The drawing under review shows one solid part. Ordinate dimensions are in mm from its lowest x, y, z. A direction names the side the tool comes from. Give positions to 0.01 mm unless a question says otherwise; leave off trailing zeros. Order: outer loops, then holes, each group sorted by start corner. A loop starts at its lowest first (then second) coordinate and runs counter-clockwise, first axis right, second up. Notation, with made-up numbers: (88, 46.25) -> (110, 46.25) arc R20 cw to (110, 68.25) -> close; hole circle Ø3 at (-24, 78). An arc over 180 degrees is marked (long way). Return JSON: item names as keys, results as strings. Group by question number.
1) The part is to be moulded in two halves that separate along X. For the marked faces 3, 4, 5 and 6, say which applies: released by +X, released by -X, zero draft, split by the parting line, or undercut.
2) Add section A-A (x = 67.5). Give the boundary of the cut face in (y, z).
3) Add section B-B (z = 15). Give the boundary of the cut face in (x, y), then the cut area to 3 significant figures.
4) Add section D-D (z = 40). Give the boundary of the cut face in (x, y).
5) Insertion check: P1, Ø24, axis at x = 47.5, z = 28, coming from the -Y side; P2, Ø3, axis at x = 52.5, y = 20, coming from the +Z side; P3, Ø12, axis at x = 25.5, y = 46.5, coming from the +Z side. Each pin has a flat end and moves straight along its axis. Give the tip position at first contact, or say it passes through.
6) Add section C-C (y = 20). Give the boundary of the cut face in (x, z).
7) For the marked faces 1 and 2, list the 3-axis set-ups (+Z, -Z, +X, -X, +Y, -Y) from which the entire face can be reached by the end or side of a thin tool; tool diameter is ignored.
8) To check wall thickness, follow line 1 along X through (y, z) = (50.5, 38.5); line 2 along Y through (x, z) = (67.5, 0.4); line 3 along Z through (x, y) = (5.5, 55). State the ranges of each line that lie inside material, in increasing order.
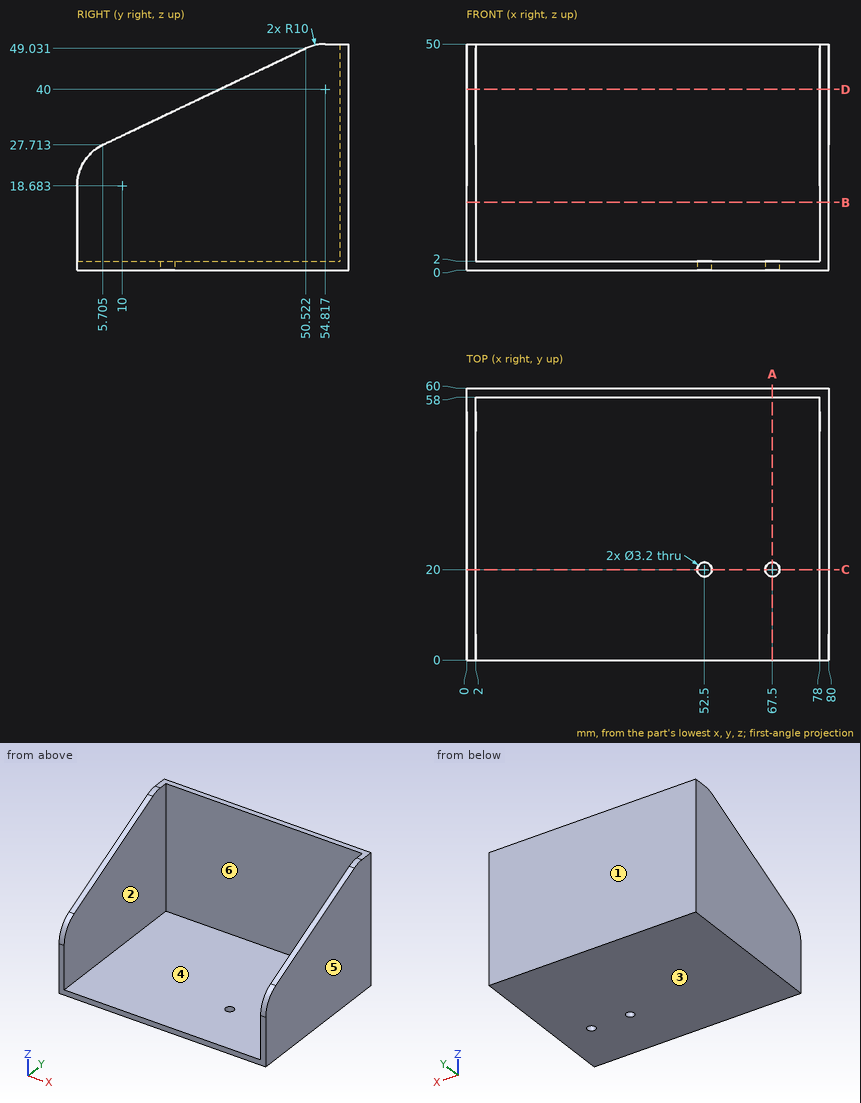
Evaluation:
{
 "1": {"face 3": "zero draft", "face 4": "undercut", "face 5": "released by +X", "face 6": "undercut"},
 "2": {"outline": "(0, 0) -> (18.4, 0) -> (18.4, 2) -> (0, 2) -> close; (21.6, 0) -> (60, 0) -> (60, 50) -> (58, 50) -> (58, 2) -> (21.6, 2) -> close"},
 "3": {"outline": "(0, 0) -> (2, 0) -> (2, 58) -> (78, 58) -> (78, 0) -> (80, 0) -> (80, 60) -> (0, 60) -> close", "area": "392 mm^2"},
 "4": {"outline": "(0, 31.54) -> (2, 31.54) -> (2, 58) -> (78, 58) -> (78, 31.54) -> (80, 31.54) -> (80, 60) -> (0, 60) -> close"},
 "5": {"P1": "y = 58", "P2": "through", "P3": "z = 2"},
 "6": {"outline": "(0, 0) -> (50.9, 0) -> (50.9, 2) -> (2, 2) -> (2, 34.51) -> (0, 34.51) -> close; (54.1, 0) -> (65.9, 0) -> (65.9, 2) -> (54.1, 2) -> close; (69.1, 0) -> (80, 0) -> (80, 34.51) -> (78, 34.51) -> (78, 2) -> (69.1, 2) -> close"},
 "7": {"face 1": "+Z, -Z, +X, -X, +Y", "face 2": "+Z, -Y"},
 "8": {"line 1": "0 to 2, 78 to 80", "line 2": "0 to 18.4, 21.6 to 60", "line 3": "0 to 2"}
}
